For this review, take the finished solid that the model builds, in its own axes (mm). A direction names the side the tool comes from. Round coordinates to 2 decimals unless told otherwise and drop trailing zeros. Loops run counter-clockwise (first coordinate to the right, second up) from the corner with the lowest first, then second, coordinate; pieces in that order, holes last. Notation, with made-up numbers: (67.5, 56) -> (72.5, 56) arc R11 ccw to (72.5, 61) -> close; hole circle Ø2 at (7.5, 37.5). An arc over 180 degrees is marked (long way). One line per question, with ' | ' between items. Start each with the question number.
1. Wall thickness on line 1 along Y through (x, z) = (-205, 456); line 2 along Y through (x, z) = (-731.5, 522); line 3 along Z through (x, y) = (-657, -53): over which ranges is each line inside the solid? List them lowest first.
2. For faces 1 (the face through (-467, -75.756, 539)), 2 (the face through (-467, -75.756, -46)), 3 (the face through (-938.545, -38, 243)), list the 3-axis set-ups (+Z, -Z, +X, -X, +Y, -Y) from which the entire face can be reached by the end or side of a thin tool; tool diameter is ignored.
3. Consider section B-B (y = -17). Write out the cut boundary in (x, z), and give its area (3 significant figures).
4. For pin 1 Ø6 at (x, z) = (-418.5, 256) entering from +Y; pin 2 Ø1.3 at (y, z) = (-77, 551.5) entering from -X; pin 3 Ø4 at (x, z) = (-387.52, 548.41) entering from +Y; pin 4 Ø19 at (x, z) = (-490.5, -47) entering from +Y, all flat-tipped, find the tip position at first contact; note any pin that passes through.
5. Consider section A-A (x = -797). Write out the cut boundary in (y, z).
6. Consider section C-C (x = -289.5). Write out the cut boundary in (y, z).
```python
from build123d import *

# Parameters (mm, degrees)
F0_W     = 952.1952
F0_H     = 545.7952
F1_DEPTH = 77.343
F2_R     = 3.175
F3_DEPTH = 1.5875
F6_W     = 930.2496
F6_H     = 523.2654
F7_DEPTH = 0.254


with BuildPart() as f1:
    # F0 (on Front) → F1 (new body)
    with BuildSketch(Plane.XZ):
        with Locations((-462.4471531919, 246.4511793006)):
            Rectangle(F0_W, F0_H)
    extrude(amount=F1_DEPTH)

    # F2 (on face) → F3 (join)
    with BuildSketch(Plane.XZ.offset(77.343)):
        with BuildLine():
            Line((-765.6215531919, 557.7789793006), (-786.2971531919, 557.7789793006))
            Line((-786.2971531919, 557.7789793006), (-786.2971531919, 519.3487793006))
            Line((-786.2971531919, 519.3487793006), (-138.5971531919, 519.3487793006))
            Line((-138.5971531919, 519.3487793006), (-138.5971531919, 557.7789793006))
            Line((-138.5971531919, 557.7789793006), (-159.2727531919, 557.7789793006))
            Line((-159.2727531919, 557.7789793006), (-159.2727531919, 548.4063793006))
            ThreePointArc((-159.2727531919, 548.4063793006), (-162.4477531919, 545.2313793006), (-165.6227531919, 548.4063793006))
            Line((-165.6227531919, 548.4063793006), (-165.6227531919, 557.7789793006))
            Line((-165.6227531919, 557.7789793006), (-462.4471531919, 557.7789793006))
            Line((-462.4471531919, 557.7789793006), (-462.4471531919, 551.5813793006))
            ThreePointArc((-462.4471531919, 551.5813793006), (-460.2020891616, 550.6514433309), (-459.2721531919, 548.4063793006))
            ThreePointArc((-459.2721531919, 548.4063793006), (-462.4471531919, 545.2313793006), (-465.6221531919, 548.4063793006))
            Line((-465.6221531919, 548.4063793006), (-534.2021531919, 548.4063793006))
            ThreePointArc((-534.2021531919, 548.4063793006), (-537.3771531919, 545.2313793006), (-540.5521531919, 548.4063793006))
            Line((-540.5521531919, 548.4063793006), (-609.2845531919, 548.4063793006))
            ThreePointArc((-609.2845531919, 548.4063793006), (-612.4595531919, 545.2313793006), (-615.6345531919, 548.4063793006))
            Line((-615.6345531919, 548.4063793006), (-684.2907531919, 548.4063793006))
            ThreePointArc((-684.2907531919, 548.4063793006), (-687.4657531919, 545.2313793006), (-690.6407531919, 548.4063793006))
            Line((-690.6407531919, 548.4063793006), (-759.2715531919, 548.4063793006))
            ThreePointArc((-759.2715531919, 548.4063793006), (-762.4465531919, 545.2313793006), (-765.6215531919, 548.4063793006))
            Line((-765.6215531919, 548.4063793006), (-765.6215531919, 557.7789793006))
        make_face()
        with Locations((-387.5171531919, 548.4063793006)):
            Circle(F2_R, mode=Mode.SUBTRACT)
        with Locations((-312.4347531919, 548.4063793006)):
            Circle(F2_R, mode=Mode.SUBTRACT)
        with Locations((-237.4285531919, 548.4063793006)):
            Circle(F2_R, mode=Mode.SUBTRACT)
        with BuildLine():
            Line((-462.4471531919, 557.7789793006), (-759.2715531919, 557.7789793006))
            Line((-759.2715531919, 557.7789793006), (-759.2715531919, 548.4063793006))
            Line((-759.2715531919, 548.4063793006), (-690.6407531919, 548.4063793006))
            ThreePointArc((-690.6407531919, 548.4063793006), (-687.4657531919, 551.5813793006), (-684.2907531919, 548.4063793006))
            Line((-684.2907531919, 548.4063793006), (-615.6345531919, 548.4063793006))
            ThreePointArc((-615.6345531919, 548.4063793006), (-612.4595531919, 551.5813793006), (-609.2845531919, 548.4063793006))
            Line((-609.2845531919, 548.4063793006), (-540.5521531919, 548.4063793006))
            ThreePointArc((-540.5521531919, 548.4063793006), (-537.3771531919, 551.5813793006), (-534.2021531919, 548.4063793006))
            Line((-534.2021531919, 548.4063793006), (-465.6221531919, 548.4063793006))
            ThreePointArc((-465.6221531919, 548.4063793006), (-464.6922172221, 550.6514433309), (-462.4471531919, 551.5813793006))
            Line((-462.4471531919, 551.5813793006), (-462.4471531919, 557.7789793006))
        make_face()
    extrude(amount=-F3_DEPTH)

    # F5: F1 across plane


with BuildPart() as f1_1:
    add(f1.part)
    add(f1.part.mirror(Plane(origin=(-462.4471531919, -38.6715, 246.4511793006), x_dir=(1, 0, 0), z_dir=(0, 0, -1))))

    # F6 (on face) → F7 (cut)
    with BuildSketch(Plane.XZ.offset(77.343)):
        with Locations((-462.4471531919, 246.4511793006)):
            Rectangle(F6_W, F6_H)
    extrude(amount=-F7_DEPTH, mode=Mode.SUBTRACT)


solid = f1_1.part
```
Answer block:
1) line 1: y = -77.09 to 0 | line 2: y = -77.34 to -75.76 | line 3: z = -26.45 to 519.35
2) face 1: +Z, +X, -X, +Y | face 2: -Z, +X, -X, +Y | face 3: +Z, -Z, -X, +Y, -Y
3) outline: (-938.54, -26.45) -> (13.65, -26.45) -> (13.65, 519.35) -> (-938.54, 519.35) -> close | area: 520,000 mm2
4) pin 1: stops at y = 0 | pin 2: stops at x = -786.3 | pin 3: passes through | pin 4: stops at y = -75.76
5) outline: (-77.34, -26.45) -> (0, -26.45) -> (0, 519.35) -> (-77.34, 519.35) -> (-77.34, 508.08) -> (-77.09, 508.08) -> (-77.09, -15.18) -> (-77.34, -15.18) -> close
6) outline: (-77.34, -64.88) -> (-75.76, -64.88) -> (-75.76, -26.45) -> (0, -26.45) -> (0, 519.35) -> (-75.76, 519.35) -> (-75.76, 557.78) -> (-77.34, 557.78) -> (-77.34, 508.08) -> (-77.09, 508.08) -> (-77.09, -15.18) -> (-77.34, -15.18) -> close
